from build123d import *

# Parameters (mm, degrees)
BASPROSKE_W        = 3.3
BASPROSKE_H        = 4.5
TOOTHCUT_DEPTH     = 8.168681887
TEETHCUTS_COUNT    = 16
TEETHCUTS_ANGLE    = 337.5
BORSKE_R           = 1.5
BORE_DEPTH         = 50.0000508
BOSS_EXTRU_1_START = 3.7
ESQUISSE1_R        = 3.17
ESQUISSE1_R_2      = 1.5
BOSS_EXTRU_1_DEPTH = 3.7


with BuildPart() as part:
    # BasProSke → Base-Revolve (revolve)
    with BuildSketch(Plane(origin=(0, 0, 0), x_dir=(1, 0, 0), z_dir=(0, 1, 0)), mode=Mode.PRIVATE) as base_revolve_sk:
        with Locations((1.65, 2.25)):
            Rectangle(BASPROSKE_W, BASPROSKE_H)
    revolve(base_revolve_sk.sketch.rotate(Axis((-10, 0, 0), (1, 0, 0)), 180), axis=Axis((-10, 0, 0), (1, 0, 0)))

    # TooCutSke → ToothCut (cut, through all)
    with BuildSketch(Plane(origin=(0, 0, 0), x_dir=(0, 0, -1), z_dir=(1, 0, 0))):
        with BuildLine():
            ThreePointArc((0.261866103, 3.363822549), (0, 3.374), (-0.261866103, 3.363822549))
            ThreePointArc((-0.261866103, 3.363822549), (-0.417714668, 3.961827375), (-0.788562282, 4.456165918))
            ThreePointArc((-0.788562282, 4.456165918), (0, 4.5254), (0.788562282, 4.456165918))
            ThreePointArc((0.788562282, 4.456165918), (0.417714668, 3.961827375), (0.261866103, 3.363822549))
        make_face()
    toothcut = extrude(amount=TOOTHCUT_DEPTH, mode=Mode.SUBTRACT)

    # TeethCuts: ToothCut ×16 about axis
    teethcuts_axis = Axis((-10, 0, 0), (1, 0, 0))
    for i in range(1, TEETHCUTS_COUNT):
        add(toothcut.rotate(teethcuts_axis, i * TEETHCUTS_ANGLE / (TEETHCUTS_COUNT - 1)), mode=Mode.SUBTRACT)

    # BorSke → Bore (cut, symmetric)
    with BuildSketch(Plane(origin=(0, 0, 0), x_dir=(0, 0, -1), z_dir=(1, 0, 0))):
        with Locations(Location((0, 0, 0), (0, 0, 180))):
            Circle(BORSKE_R)
    extrude(amount=BORE_DEPTH, both=True, mode=Mode.SUBTRACT)

    # Esquisse1 → Boss.-Extru.1 (add)
    with BuildSketch(Plane(origin=(3.3, 0, 0), x_dir=(0, 0, -1), z_dir=(1, 0, 0)).offset(BOSS_EXTRU_1_START)):
        with Locations(Location((0, 0, 0), (0, 0, 180))):
            Circle(ESQUISSE1_R)
        Circle(ESQUISSE1_R_2, mode=Mode.SUBTRACT)
    extrude(amount=-BOSS_EXTRU_1_DEPTH)


solid = part.part
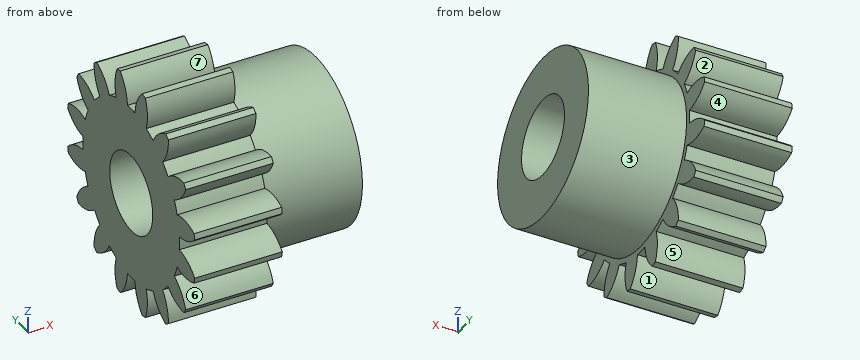
For this review, take the finished solid that the model builds, in its own axes (mm). Face numbers are marked on the shaded views. A direction names the side the tool comes from. Coordinates: 2 decimals unless noted, no trailing zeros. Order: outer loops, then holes, each group sorted by start corner. A loop starts at its lowest first (then second) coordinate and runs counter-clockwise, first axis right, second up. Notation, with made-up numbers: (-7.5, 23.25) - (2.5, 23.25) arc R10 cw to (2.5, 40.25) - close; hole circle Ø5 at (87, 67.25). An arc over 180 degrees is marked (long way). Answer as CSV lines item,"result". Start each with the question number.
1) Add section C-C (x = 6.5). State the section outline as (y, z) points, then the cut area to 3 significant figures.
2) Machinability: for the marked faces 4, 5, 6 and 7, which of the approach directions +Z, -Z, +X, -X, +Y, -Y give a long, thin tool a straight path to every point of the face, cutting with its end or side? Answer none if there is none.
3) Insertion check: P1, Ø2, axis at x = 5, y = 0.5, coming from the -Z side; P2, Ø4, axis at x = 6, z = -3, coming from the +Y side; P3, Ø1, axis at x = 4.5, y = -2, coming from the -Z side. Each pin has a flat end and moves straight along its axis. Give the tip position at first contact, or say it passes through.
4) Draft analysis for pull direction Y (two halves, no side actions). For the marked faces 1, 2 and 3, state which applies: +Y half, -Y half, draft (parallel to the pull), parting line (faces both ways), or undercut.
5) To check wall thickness, follow line 1 along Y through (x, z) = (4, 0); line 2 along Y through (x, z) = (2.75, 0); line 3 along Y through (x, z) = (3.25, 3.5). State the ranges of each line that lie inside material, in increasing order. Write a range as [from, to].
6) Add section D-D (y = 3.5). State the section outline as (x, z) points.
7) Add section A-A (z = 0). State the section outline as (x, y) points, then the cut area to 3 significant figures.
Result:
1,outline,"circle Ø6.34 at (0, 0); hole circle Ø3 at (0, 0)"
1,area,"24.5 mm^2"
2,face 4,"+X, -X, +Y"
2,face 5,"+X, -X"
2,face 6,"+X, -X, -Y"
2,face 7,"+Z, +X, -X"
3,P1,"z = -3.17"
3,P2,"y = 3.01"
3,P3,"z = -2.79"
4,face 1,"undercut"
4,face 2,"+Y half"
4,face 3,"parting line"
5,line 1,"[-3.17, -1.5], [1.5, 3.17]"
5,line 2,"[-3.37, -1.5], [1.5, 3.37]"
5,line 3,"[-2.59, -1.9], [-1.12, -0.28], [0.28, 1.12], [1.9, 2.59]"
6,outline,"(0, -2.59) - (3.3, -2.59) - (3.3, -1.9) - (0, -1.9) - close; (0, -1.12) - (3.3, -1.12) - (3.3, -0.28) - (0, -0.28) - close; (0, 0.28) - (3.3, 0.28) - (3.3, 1.12) - (0, 1.12) - close; (0, 1.9) - (3.3, 1.9) - (3.3, 2.59) - (0, 2.59) - close"
7,outline,"(0, -3.37) - (3.3, -3.37) - (3.3, -3.17) - (7, -3.17) - (7, -1.5) - (0, -1.5) - close; (0, 1.5) - (7, 1.5) - (7, 3.17) - (3.3, 3.17) - (3.3, 3.37) - (0, 3.37) - close"
7,area,"24.7 mm^2"
